```python
from build123d import *

# Parameters (mm, degrees)
SKETCH_W        = 40
SKETCH_H        = 11
PAD_DEPTH       = 4.75
SKETCH001_W     = 40
SKETCH001_H     = 1.75
POCKET_DEPTH    = 8
SKETCH002_W     = 8
SKETCH002_H     = 3
PAD001_DEPTH    = 8
SKETCH004_R     = 1.6
POCKET001_DEPTH = 11.001
FILLET_R        = 1


with BuildPart() as part:
    # Sketch → Pad (new body)
    with BuildSketch(Plane.XY):
        with Locations((0, -2.5)):
            Rectangle(SKETCH_W, SKETCH_H)
    extrude(amount=PAD_DEPTH)

    # Sketch001 (on Face3 of Pad) → Pocket (cut)
    with BuildSketch(Plane.XZ.offset(8)):
        with Locations((0, 2.375)):
            Rectangle(SKETCH001_W, SKETCH001_H)
    extrude(amount=-POCKET_DEPTH, mode=Mode.SUBTRACT)

    # Sketch002 (on Face5 of Pocket) → Pad001 (join)
    with BuildSketch(Plane.XY.offset(4.75)):
        with Locations((-16, 1.5)):
            Rectangle(SKETCH002_W, SKETCH002_H)
        with Locations((16, 1.5)):
            Rectangle(SKETCH002_W, SKETCH002_H)
    extrude(amount=PAD001_DEPTH)

    # Sketch004 (on Face7 of Pad001) → Pocket001 (cut, through all)
    with BuildSketch(Plane(origin=(0, 3, 0), x_dir=(-1, 0, 0), z_dir=(0, 1, 0))):
        with Locations((-16, 8.75)):
            Circle(SKETCH004_R)
        with Locations((16, 8.75)):
            Circle(SKETCH004_R)
    extrude(amount=-POCKET001_DEPTH, mode=Mode.SUBTRACT)

    # Fillet
    fillet_edges = [part.edges().sort_by_distance(p)[0] for p in [
        (20, 1.5, 12.75),
        (12, 1.5, 12.75),
        (-12, 1.5, 12.75),
        (-20, 1.5, 12.75),
    ]]
    fillet(fillet_edges, radius=FILLET_R)


solid = part.part
```
The model under review builds one solid part; all positions refer to its coordinate system, in mm. A direction names the side the tool comes from. Give positions to 0.01 mm unless a question says otherwise; leave off trailing zeros. Write each loop counter-clockwise with the first axis right and the second up, starting at its lowest first coordinate (ties: lowest second). Pieces come first, ordered by that corner, then holes. Notation, with made-up numbers: M 20,-19.5 L 56,-19.5 A13 cw 56,-3.5 Z; hole C 25.5,41.5 d4. An arc over 180 degrees is marked long. Answer in a Markdown table with one row per item.
Item 1: Tool access review of faces 1 (the face through (18, 0, 9)), 2 (the face through (12, 1, 8)), 3 (the face through (0, -4, 1.5)): name each direction out of +Z, -Z, +X, -X, +Y, -Y from which nothing blocks a thin tool from reaching the whole face with its end or side.
Check sheet entries:
| item | result |
|---|---|
| face 1 | +Z, +X, -X, -Y |
| face 2 | +Z, +Y, -Y |
| face 3 | +X, -X, -Y |
Item 2: Draft analysis for pull direction X (two halves, no side actions). For faces 4 (the face through (20, 0, 4)), 5 (the face through (0, -4, 4.75)), 6 (the face through (0, -8, 4)), state which applies: +X half, -X half, draft (parallel to the pull), parting line (faces both ways), or undercut.
Check sheet entries:
| item | result |
|---|---|
| face 4 | +X half |
| face 5 | undercut |
| face 6 | draft |
Item 3: Add section C-C on x = -16. Give the boundary of the cut face in (y, z).
Check sheet entries:
| item | result |
|---|---|
| outline | M -8,0 L 3,0 L 3,7.15 L 0,7.15 L 0,4.75 L -8,4.75 L -8,3.25 L 0,3.25 L 0,1.5 L -8,1.5 Z; M 0,10.35 L 3,10.35 L 3,12.75 L 0,12.75 Z |
Item 4: For line 1 along X through (y, z) = (1.75, 6.75); line 2 along Z through (x, y) = (1.5, -6.25); line 3 along Z through (x, y) = (16, 1.1), list the stretches that pass through material, from the lowest coordinate up.
Check sheet entries:
| item | result |
|---|---|
| line 1 | -20 to -12, 12 to 20 |
| line 2 | 0 to 1.5, 3.25 to 4.75 |
| line 3 | 0 to 7.15, 10.35 to 12.75 |
Item 5: Add section A-A on y = -2. Give the boundary of the cut face in (x, z), plus the area to 3 significant figures.
Check sheet entries:
| item | result |
|---|---|
| outline | M -20,0 L 20,0 L 20,1.5 L -20,1.5 Z; M -20,3.25 L 20,3.25 L 20,4.75 L -20,4.75 Z |
| area | 120 mm2 |
Item 6: Add section B-B on z = 5.5. Give the boundary of the cut face in (x, y), plus the area to 3 significant figures.
Check sheet entries:
| item | result |
|---|---|
| outline | M -20,0 L -12,0 L -12,3 L -20,3 Z; M 12,0 L 20,0 L 20,3 L 12,3 Z |
| area | 48.0 mm2 |
Item 7: For P1, Ø3, axis at y = -2.5, z = 10.5, coming from the +X side; P2, Ø6.5, axis at x = -15, z = 8.5, coming from the -Y side; P3, Ø5, axis at x = -16, z = 8.75, coming from the +Y side; P4, Ø4, axis at x = -6, y = -1, coming from the +Z side, all flat-tipped, find the tip position at first contact; note any pin that passes through.
Check sheet entries:
| item | result |
|---|---|
| P1 | through |
| P2 | y = 0 |
| P3 | y = 3 |
| P4 | z = 4.75 |
Item 8: Add section D-D on z = 8.75. Give the boundary of the cut face in (x, y), plus the area to 3 significant figures.
Check sheet entries:
| item | result |
|---|---|
| outline | M -20,0 L -17.6,0 L -17.6,3 L -20,3 Z; M -14.4,0 L -12,0 L -12,3 L -14.4,3 Z; M 12,0 L 14.4,0 L 14.4,3 L 12,3 Z; M 17.6,0 L 20,0 L 20,3 L 17.6,3 Z |
| area | 28.8 mm2 |
